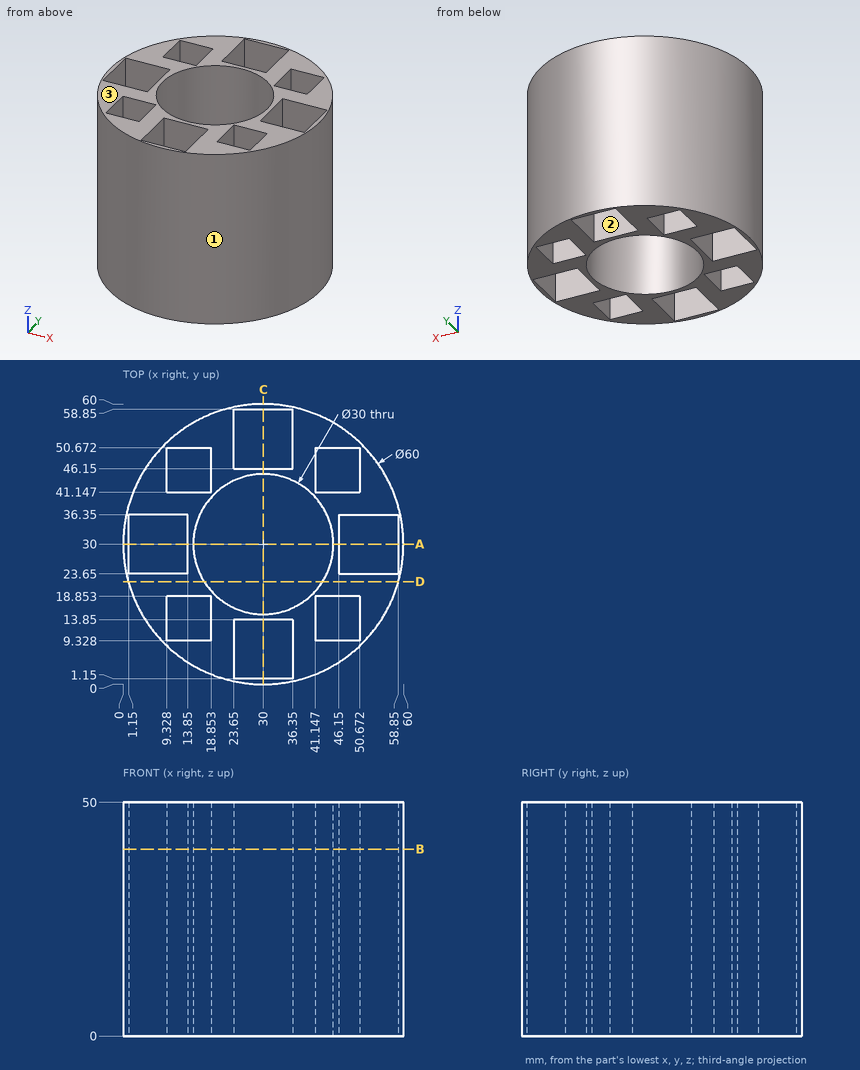
For this review, use the dimensioned drawing (mm, ordinates from the lowest corner) and the shaded views. Round coordinates to 2 decimals unless told otherwise and drop trailing zeros. Order: outer loops, then holes, each group sorted by start corner. A loop starts at its lowest first (then second) coordinate and runs counter-clockwise, first axis right, second up. Notation, with made-up numbers: M -31,85.25 L 12,85.25 A29 ccw 12,108.25 Z; hole C 4.5,84 d2. An arc over 180 degrees is marked long. Use a Markdown table: item, result. Add a question column.
Item 1: Insertion check: pin 1 (7.5 mm diameter, centred on y = 45, z = 23, fed in from +X); pin 2 (6 mm diameter, centred on x = 27.5, z = 11, fed in from -Y); pin 3 (10 mm diameter, centred on x = 52, z = 5.5, fed in from -Y). Each pin has a flat end and moves straight along its axis. Give the tip position at first contact, or say it passes through.
Item 2: Add section B-B, the plane z = 40. State how many separate pieces and enclosed holes the cut face has, then the cut area to 3 significant figures.
Item 3: To check wall thickness, follow line 1 along Y through (x, z) = (30, 11.5); line 2 along Y through (x, z) = (45.5, 20) (1 decimal). State the ranges of each line that lie inside material, in increasing order.
Item 4: Add section A-A, the plane y = 30. Give the boundary of the cut face in (x, z), then the cut area to 3 significant figures.
Item 5: Mouldability with a two-part tool opening along X and no side actions: class the marked faces 1, 2 and 3 as released by +X, released by -X, zero draft, split by the parting line, or undercut.
Item 6: Add section D-D, the plane y = 22. Give the boundary of the cut face in (x, z).
Geometry results:
| question | item | result |
|---|---|---|
| 1 | pin 1 | stops at x = 57.81 |
| 1 | pin 2 | stops at y = 0 |
| 1 | pin 3 | stops at y = 5.28 |
| 2 | separate pieces | 1 |
| 2 | enclosed holes | 9 |
| 2 | area | 1,110 mm² |
| 3 | line 1 | y = 0 to 1.15, 13.85 to 15, 45 to 46.15, 58.85 to 60 |
| 3 | line 2 | y = 4.3 to 9.3, 18.9 to 41.1, 50.7 to 55.7 |
| 4 | outline | M 0,0 L 1.15,0 L 1.15,50 L 0,50 Z; M 13.85,0 L 15,0 L 15,50 L 13.85,50 Z; M 45,0 L 46.15,0 L 46.15,50 L 45,50 Z; M 58.85,0 L 60,0 L 60,50 L 58.85,50 Z |
| 4 | area | 230 mm² |
| 5 | face 1 | split by the parting line |
| 5 | face 2 | undercut |
| 5 | face 3 | zero draft |
| 6 | outline | M 1.09,0 L 17.31,0 L 17.31,50 L 1.09,50 Z; M 42.69,0 L 58.91,0 L 58.91,50 L 42.69,50 Z |
